For this review, take the finished solid that the model builds, in its own axes (mm). Give positions to 0.01 mm unless a question says otherwise; leave off trailing zeros. Order: outer loops, then holes, each group sorted by start corner. A loop starts at its lowest first (then second) coordinate and runs counter-clockwise, first axis right, second up.
Item 1: The part is to be moulded in two halves that separate along X. For faces 1 (the flat face through (9.442, 0.049, 5.554)), 2 (the flat face through (7, 3.937, 2)), 3 (the cylindrical face through (-6.834, -0.055, -1.517)), say which applies: released by +X, released by -X, zero draft, split by the parting line, or undercut.
Item 2: Consider section A-A (y = 1). Give the boundary of the cut face in (x, z).
Item 3: For P1, Ø2, axis at y = 2, z = 1.5, coming from the -X side, flat-tipped, find the tip position at first contact; note if it passes through.
Item 4: For probe 1 along X at (y, z) = (-3, -5.25); probe 2 along X at (y, z) = (2.5, 2); probe 3 along Z at (x, y) = (0.75, -1), list the stretches that pass through material, from the lowest coordinate up.
```python
from build123d import *

# Parameters (mm, degrees)
SKETCH1_R           = 7
BOSS_EXTRUDE1_DEPTH = 3.937


# Read off the part's stored shape, not the designer's step: Cut-Revolve-Thin1
with BuildPart() as part:
    # Sketch1 → Boss-Extrude1 (new, symmetric)
    with BuildSketch(Plane(origin=(0, 0, 0), x_dir=(1, 0, 0), z_dir=(0, 1, 0))):
        Polygon((6.324150511, 10.95375), (-6.324150511, 10.95375), (-12.648301022, 0), (-6.324150511, -10.95375), (6.324150511, -10.95375), (12.648301022, 0), align=None)
        with Locations(Location((0, 0, 0), (0, 0, 270))):
            Circle(SKETCH1_R, mode=Mode.SUBTRACT)
    extrude(amount=BOSS_EXTRUDE1_DEPTH, both=True)

    # Cut-Revolve-Thin1 outline → Cut-Revolve-Thin1 (revolve, cut)
    with BuildSketch(Plane.XY):
        with BuildLine():
            ThreePointArc((12.648306093, -1.426964265), (11.685557296, -2.803541534), (10.44575, -3.937))
            Line((10.44575, -3.937), (12.648306093, -3.937))
            Line((12.648306093, -3.937), (12.648306093, -1.426964265))
        make_face()
        with BuildLine():
            ThreePointArc((10.44575, 3.937), (11.685557296, 2.803541534), (12.648306093, 1.426964265))
            Line((12.648306093, 1.426964265), (12.648306093, 3.937))
            Line((12.648306093, 3.937), (10.44575, 3.937))
        make_face()
    revolve(axis=Axis((0, 0, 0), (0, 1, 0)), mode=Mode.SUBTRACT)


solid = part.part
```
Resolved:
1. face 1: released by +X
1. face 2: zero draft
1. face 3: undercut
2. outline: (-12.65, 0) - (-6.32, -10.95) - (6.32, -10.95) - (12.65, 0) - (6.32, 10.95) - (-6.32, 10.95) - close; hole circle Ø14 at (0, 0)
3. P1: stops at x = -12.36
4. probe 1: x = -9.62 to -4.63, 4.63 to 9.62
4. probe 2: x = -11.49 to -6.71, 6.71 to 11.49
4. probe 3: z = -10.95 to -6.96, 6.96 to 10.95
